Here's how the part is built. I have some questions about the finished solid (model axes, mm). A direction names the side the tool comes from. Round coordinates to 2 decimals unless told otherwise and drop trailing zeros. Write each loop counter-clockwise with the first axis right and the second up, starting at its lowest first coordinate (ties: lowest second). Pieces come first, ordered by that corner, then holes. Notation, with made-up numbers: (88, 86) -> (114, 86) arc R21 ccw to (114, 92) -> close; hole circle Ø11 at (63.25, -38). An arc over 180 degrees is marked (long way). Put each result on its own line as item: value. Start each with the question number.
1) If I drill on line 1 along X through (y, z) = (-0.5, 9.5); line 2 along X through (y, z) = (-0.8, -5); line 3 along Z through (x, y) = (3, -0.9), over which ranges is the centre line in solid material (lowest first)? Write a range as [from, to].
2) I want a section at C-C, the plane x = -2.25. List the corners of the cut face in (y, z) for me.
3) Will this pin go through, and if not, where does the flat tip stop? P1, Ø5, axis at x = -3, z = -6.5, coming from the -Y side.
4) I want a section at A-A, the plane z = 7.5. List the corners of the cut face in (x, y) for me.
5) We'd pull the mould along Z, two halves only. Please class faces 1 (the flat face through (-3.5, -0.5, 10)), 2 (the flat face through (0, -1, 0)), 3 (the flat face through (-0.1, -0.5, 11)): released by +Z, released by -Z, zero draft, split by the parting line, or undercut.
6) I want a section at D-D, the plane z = 3.5. List the corners of the cut face in (x, y) for me.
7) I want a section at B-B, the plane y = -0.15. List the corners of the cut face in (x, z) for me, then the cut area to 3 significant figures.
8) Which directions (+Z, -Z, +X, -X, +Y, -Y) give clear straight access to the entire face, cutting with the end or side of a thin tool? Please do faces 4 (the flat face through (6, -0.5, -0.2)), 5 (the flat face through (3, -0.5, 1)), 6 (the flat face through (3.5, -0.5, 5)).
from build123d import *

# Parameters (mm, degrees)
SKETCH_W        = 12
SKETCH_H        = 22
PAD_DEPTH       = 1
SKETCH001_W     = 4.5
SKETCH001_H     = 6.5
POCKET_DEPTH    = 0.5
SKETCH002_W     = 3
SKETCH002_H     = 5
POCKET001_DEPTH = 5


with BuildPart() as part:
    # Sketch → Pad (new body)
    with BuildSketch(Plane.XZ):
        Rectangle(SKETCH_W, SKETCH_H)
    extrude(amount=PAD_DEPTH)

    # Sketch001 (on Face6 of Pad) → Pocket (cut)
    with BuildSketch(Plane.XZ.offset(1)):
        with Locations((-2.75, -6.75)):
            Rectangle(SKETCH001_W, SKETCH001_H)
        with Locations((2.75, -6.75)):
            Rectangle(SKETCH001_W, SKETCH001_H)
        with Locations((-2.75, 0.75)):
            Rectangle(SKETCH001_W, SKETCH001_H)
        with Locations((2.75, 0.75)):
            Rectangle(SKETCH001_W, SKETCH001_H)
    extrude(amount=-POCKET_DEPTH, mode=Mode.SUBTRACT)

    # Sketch002 (on Face5 of Pocket) → Pocket001 (cut)
    with BuildSketch(Plane.XZ.offset(1)):
        with Locations((-3.5, 7.5)):
            Rectangle(SKETCH002_W, SKETCH002_H)
        with Locations((0, 7.5)):
            Rectangle(SKETCH002_W, SKETCH002_H)
        with Locations((3.5, 7.5)):
            Rectangle(SKETCH002_W, SKETCH002_H)
    extrude(amount=-POCKET001_DEPTH, mode=Mode.SUBTRACT)


solid = part.part
Findings:
1. line 1: x = [-6, -5], [-2, -1.5], [1.5, 2], [5, 6]
1. line 2: x = [-6, -5], [-0.5, 0.5], [5, 6]
1. line 3: z = [-11, -10], [-3.5, -2.5], [4, 5], [10, 11]
2. outline: (-1, -11) -> (0, -11) -> (0, 5) -> (-1, 5) -> (-1, 4) -> (-0.5, 4) -> (-0.5, -2.5) -> (-1, -2.5) -> (-1, -3.5) -> (-0.5, -3.5) -> (-0.5, -10) -> (-1, -10) -> close; (-1, 10) -> (0, 10) -> (0, 11) -> (-1, 11) -> close
3. P1: stops at y = -1
4. outline: (-6, -1) -> (-5, -1) -> (-5, 0) -> (-6, 0) -> close; (-2, -1) -> (-1.5, -1) -> (-1.5, 0) -> (-2, 0) -> close; (1.5, -1) -> (2, -1) -> (2, 0) -> (1.5, 0) -> close; (5, -1) -> (6, -1) -> (6, 0) -> (5, 0) -> close
5. face 1: undercut
5. face 2: zero draft
5. face 3: released by +Z
6. outline: (-6, -1) -> (-5, -1) -> (-5, -0.5) -> (-0.5, -0.5) -> (-0.5, -1) -> (0.5, -1) -> (0.5, -0.5) -> (5, -0.5) -> (5, -1) -> (6, -1) -> (6, 0) -> (-6, 0) -> close
7. outline: (-6, -11) -> (6, -11) -> (6, 11) -> (-6, 11) -> close; hole (-5, 5) -> (-2, 5) -> (-2, 10) -> (-5, 10) -> close; hole (-1.5, 5) -> (1.5, 5) -> (1.5, 10) -> (-1.5, 10) -> close; hole (2, 5) -> (5, 5) -> (5, 10) -> (2, 10) -> close
7. area: 219 mm2
8. face 4: +Z, -Z, +X, +Y, -Y
8. face 5: -Y
8. face 6: +Y, -Y
